Input: part model. Units: mm. Frame: model coordinates. A direction names the side the tool comes from. Coordinates: 2 decimals unless noted, no trailing zeros. Loops run counter-clockwise (first coordinate to the right, second up) from the corner with the lowest first, then second, coordinate; pieces in that order, holes last.
(1) Section C-C, the plane y = 8. Return loops of the section in (x, z), then the cut area to 3 significant figures.
(2) Section A-A, the plane x = 0. Return loops of the section in (y, z).
(3) Contact query for flat-ended pins moving along their axis: P1, Ø8, axis at x = -27, y = 22, coming from the +Z side; P2, Ø5, axis at y = 13, z = -41.5, coming from the +X side; P3, Ø4, axis at y = 4, z = -41, coming from the -X side. Output: stop coordinate, or through.
(4) Line query: L1, parallel to Z at x = 0.5, y = 4; L2, parallel to Z at x = 22.5, y = 8; L3, parallel to X at y = 2.25, z = 45. Output: solid intervals per line, ascending.
(5) Section B-B, the plane z = 0. Return loops of the section in (x, y).
(6) Mould query, pull axis X, two halves, no side actions, for faces 5 (the face through (4, 24.8, -42)), 6 (the face through (-11, 21.8, -41)), 7 (the face through (15.725, 21.42, 49.933)). Classes: released by +X, released by -X, zero draft, split by the parting line, or undercut.
(7) Set-up query: faces 1 (the face through (-20, 0, 49)), 2 (the face through (49, 20, 20)), 3 (the face through (49.997, 13.282, 0.508)), 4 (the face through (-16.43, 23.32, 40.44)). Return all of +Z, -Z, +X, -X, +Y, -Y with unobstructed straight access to the full face (end or side cutting, diameter ignored); none if empty.
```python
from build123d import *

# Parameters (mm, degrees)
SKETCH1_R           = 55
BOSS_EXTRUDE1_DEPTH = 24.8
SHELL1_T            = -5
SKETCH2_R           = 35
CUT_EXTRUDE1_DEPTH  = 6
SKETCH3_R           = 42
CUT_EXTRUDE2_DEPTH  = 25.8
SKETCH4_R           = 4.15
CUT_EXTRUDE3_DEPTH  = 25.8
SKETCH6_R           = 50
CUT_EXTRUDE4_DEPTH  = 2
CUT_EXTRUDE5_DEPTH  = 4
FILLET1_R           = 10
SKETCH8_OUTSIDE_W   = 143.506
SKETCH8_OUTSIDE_H   = 143.506
SKETCH8_OUTSIDE_R   = 52.35
CUT_EXTRUDE6_DEPTH  = 4.8
CHAMFER1_SIZE       = 2
CHAMFER1_SIZE2      = 1.154700538
SKETCH9_R           = 52.5
CUT_EXTRUDE7_DEPTH  = 5


with BuildPart() as part:
    # Sketch1 → Boss-Extrude1 (new body)
    with BuildSketch(Plane(origin=(0, 0, 0), x_dir=(1, 0, 0), z_dir=(0, 1, 0))):
        with Locations(Location((0, 0, 0), (0, 0, 270))):  # turned: the seam where the file's is
            Circle(SKETCH1_R)
    extrude(amount=BOSS_EXTRUDE1_DEPTH)

    # Shell1
    shell1_openings = [part.faces().sort_by_distance(p)[0] for p in [
        (0, 0, 0),
    ]]
    offset(amount=SHELL1_T, openings=shell1_openings, kind=Kind.INTERSECTION)

    # Sketch2 → Cut-Extrude1 (cut, through all)
    with BuildSketch(Plane.XZ.offset(-19.8)):
        with Locations(Location((0, 0, 0), (0, 0, 270))):  # turned: the seam where the file's is
            Circle(SKETCH2_R)
    extrude(amount=-CUT_EXTRUDE1_DEPTH, mode=Mode.SUBTRACT)

    # Sketch3 → Cut-Extrude2 (cut, through all)
    with BuildSketch(Plane(origin=(0, 24.8, 0), x_dir=(1, 0, 0), z_dir=(0, 1, 0))):
        with Locations(Location((0, 0, 0), (0, 0, 270))):  # turned: the seam where the file's is
            Circle(SKETCH3_R)
    extrude(amount=-CUT_EXTRUDE2_DEPTH, mode=Mode.SUBTRACT)

    # Sketch4 → Cut-Extrude3 (cut, through all)
    with BuildSketch(Plane(origin=(0, 24.8, 0), x_dir=(1, 0, 0), z_dir=(0, 1, 0))):
        with Locations(Location((-33.234018716, -33.234018716, 0), (0, 0, 270))):  # turned: the seam where the file's is
            Circle(SKETCH4_R)
        with Locations(Location((-33.234018716, 33.234018716, 0), (0, 0, 270))):  # turned: the seam where the file's is
            Circle(SKETCH4_R)
        with Locations(Location((33.234018716, 33.234018716, 0), (0, 0, 270))):  # turned: the seam where the file's is
            Circle(SKETCH4_R)
        with Locations(Location((33.234018716, -33.234018716, 0), (0, 0, 270))):  # turned: the seam where the file's is
            Circle(SKETCH4_R)
    extrude(amount=-CUT_EXTRUDE3_DEPTH, mode=Mode.SUBTRACT)

    # Sketch6 → Cut-Extrude4 (cut)
    with BuildSketch(Plane.XZ.offset(-19.8)):
        Circle(SKETCH6_R)
    extrude(amount=-CUT_EXTRUDE4_DEPTH, mode=Mode.SUBTRACT)

    # Sketch7 → Cut-Extrude5 (cut, through all)
    with BuildSketch(Plane.XZ.offset(-21.8)):
        with BuildLine():
            Line((15, 33.234018716), (15, 47.696960071))
            ThreePointArc((15, 47.696960071), (0, 50), (-15, 47.696960071))
            Line((-15, 47.696960071), (-15, 33.234018716))
            Line((-15, 33.234018716), (15, 33.234018716))
        make_face()
    extrude(amount=-CUT_EXTRUDE5_DEPTH, mode=Mode.SUBTRACT)

    # Fillet1
    fillet1_edges = [part.edges().sort_by_distance(p)[0] for p in [
        (-15, 23.3, 39.230090492),
        (15, 23.3, 39.230090492),
    ]]
    fillet(fillet1_edges, radius=FILLET1_R)

    # Sketch8 outside → Cut-Extrude6 (cut)
    with BuildSketch(Plane(origin=(0, 24.8, 0), x_dir=(1, 0, 0), z_dir=(0, 1, 0))):
        Rectangle(SKETCH8_OUTSIDE_W, SKETCH8_OUTSIDE_H)
        with Locations(Location((0, 0, 0), (0, 0, 270))):  # turned: the seam where the file's is
            Circle(SKETCH8_OUTSIDE_R, mode=Mode.SUBTRACT)
    extrude(amount=-CUT_EXTRUDE6_DEPTH, mode=Mode.SUBTRACT)

    # Chamfer1
    chamfer1_edges = [part.edges().sort_by_distance(p)[0] for p in [
        (0, 24.8, -52.35),
    ]]
    chamfer1_side = [part.faces().sort_by_distance(p)[0] for p in [
        (0, 22.4, -52.35),
    ]]
    chamfer(chamfer1_edges, length=CHAMFER1_SIZE, length2=CHAMFER1_SIZE2, reference=chamfer1_side[0])

    # Sketch9 → Cut-Extrude7 (cut)
    with BuildSketch(Plane.XZ):
        with Locations(Location((0, 0, 0), (0, 0, 270))):  # turned: the seam where the file's is
            Circle(SKETCH9_R)
    extrude(amount=-CUT_EXTRUDE7_DEPTH, mode=Mode.SUBTRACT)


solid = part.part
```
Report:
1. outline: circle Ø110 at (0, 0); hole (-37.38, -33.2) arc R4.15 ccw to (-33.2, -37.38) arc R50 ccw to (33.2, -37.38) arc R4.15 ccw to (37.38, -33.2) arc R50 ccw to (37.38, 33.2) arc R4.15 ccw to (33.2, 37.38) arc R50 ccw to (-33.2, 37.38) arc R4.15 ccw to (-37.38, 33.2) arc R50 ccw to start
1. area: 1,630 mm2
2. outline: (0, -55) - (20, -55) - (20, -52.35) - (22.8, -52.35) - (24.8, -51.2) - (24.8, -42) - (21.8, -42) - (21.8, -50) - (5, -50) - (5, -52.5) - (0, -52.5) - close; (0, 52.5) - (5, 52.5) - (5, 50) - (24.8, 50) - (24.8, 51.2) - (22.8, 52.35) - (20, 52.35) - (20, 55) - (0, 55) - close
3. P1: stops at z = 49.71
3. P2: stops at x = 38.78
3. P3: stops at x = -38.78
4. L1: z = -55 to -52.5, 52.5 to 55
4. L2: z = -50.19 to -44.65, 44.65 to 50.19
4. L3: x = -31.62 to -27.04, 27.04 to 31.62
5. outline: (-55, 0) - (-52.5, 0) - (-52.5, 5) - (-50, 5) - (-50, 21.8) - (-42, 21.8) - (-42, 24.8) - (-51.2, 24.8) - (-52.35, 22.8) - (-52.35, 20) - (-55, 20) - close; (42, 21.8) - (50, 21.8) - (50, 5) - (52.5, 5) - (52.5, 0) - (55, 0) - (55, 20) - (52.35, 20) - (52.35, 22.8) - (51.2, 24.8) - (42, 24.8) - close
6. face 5: zero draft
6. face 6: undercut
6. face 7: split by the parting line
7. face 1: +Z, -Z, +X, -X, -Y
7. face 2: +Y
7. face 3: -Y
7. face 4: +Y, -Y
